Work out the finished part from the listing and answer in its coordinate system (mm). Coordinates: 2 decimals unless noted, no trailing zeros. Order: outer loops, then holes, each group sorted by start corner. A loop starts at its lowest first (then second) coordinate and runs counter-clockwise, first axis right, second up.
1. The part is cut by section C-C, the plane x = -66.5. Give the vertices of the cut face in (y, z).
2. The part is cut by section B-B, the plane z = -0.45. Give the vertices of the cut face in (x, y).
3. The part is cut by section A-A, the plane y = 8. Give the vertices of the cut face in (x, z), then the cut area to 3 significant figures.
4. Find the intervals of material crossed by probe 1 along Y at (x, z) = (30, 0.25); probe 2 along Y at (x, z) = (-43.5, 0.15); probe 3 along X at (y, z) = (58.5, 0.65), in increasing order.
5. A flat-ended cylindrical pin translates along its axis: pin 1 Ø4 at (x, y) = (30, 127.5) entering from +Z. Find the tip coordinate at first contact, or state that the pin passes through.
```python
from build123d import *

# Parameters (mm, degrees)
F0_W     = 300
F0_H     = 300
F0_R     = 2.5
F0_W_2   = 100
F0_H_2   = 225
F1_DEPTH = 1


with BuildPart() as f1:
    # F0 (on Top) → F1 (new body, symmetric)
    with BuildSketch(Plane.XY):
        Rectangle(F0_W, F0_H)
        with Locations((30, -127.5)):
            Circle(F0_R, mode=Mode.SUBTRACT)
        with Locations((-30, 0)):
            Rectangle(F0_W_2, F0_H_2, mode=Mode.SUBTRACT)
        with Locations((30, 127.5)):
            Circle(F0_R, mode=Mode.SUBTRACT)
    extrude(amount=F1_DEPTH, both=True)


solid = f1.part
```
Geometry says:
1. outline: (-150, -1) - (-112.5, -1) - (-112.5, 1) - (-150, 1) - close; (112.5, -1) - (150, -1) - (150, 1) - (112.5, 1) - close
2. outline: (-150, -150) - (150, -150) - (150, 150) - (-150, 150) - close; hole (-80, -112.5) - (20, -112.5) - (20, 112.5) - (-80, 112.5) - close; hole circle Ø5 at (30, -127.5); hole circle Ø5 at (30, 127.5)
3. outline: (-150, -1) - (-80, -1) - (-80, 1) - (-150, 1) - close; (20, -1) - (150, -1) - (150, 1) - (20, 1) - close
3. area: 400 mm2
4. probe 1: y = -150 to -130, -125 to 125, 130 to 150
4. probe 2: y = -150 to -112.5, 112.5 to 150
4. probe 3: x = -150 to -80, 20 to 150
5. pin 1: passes through
